```python
from build123d import *

# Parameters (mm, degrees)
F0_W     = 117
F0_H     = 40
F0_W_2   = 2
F1_DEPTH = 1.6
F2_DEPTH = 2.8
F3_W     = 119
F3_H     = 40
F3_W_2   = 115
F3_H_2   = 38
F4_DEPTH = 1
F6_DEPTH = 2
F8_DEPTH = 2


with BuildPart() as f1:
    # F0 (on Top) → F1 (new body)
    with BuildSketch(Plane.XY):
        with BuildLine():
            Line((62.5, 26), (-62.5, 26))
            ThreePointArc((-62.5, 26), (-63.914214, 25.414214), (-64.5, 24))
            Line((-64.5, 24), (-64.5, -24))
            ThreePointArc((-64.5, -24), (-63.914214, -25.414214), (-62.5, -26))
            Line((-62.5, -26), (62.5, -26))
            ThreePointArc((62.5, -26), (63.914214, -25.414214), (64.5, -24))
            Line((64.5, -24), (64.5, 24))
            ThreePointArc((64.5, 24), (63.914214, 25.414214), (62.5, 26))
        make_face()
        Polygon((60.5, 22), (60.5, 20), (60.5, -20), (60.5, -22), (-60.5, -22), (-60.5, 22), align=None, mode=Mode.SUBTRACT)
        Polygon((-58.5, -20), (-58.5, 20), (58.5, 20), (60.5, 20), (60.5, 22), (-60.5, 22), (-60.5, -22), (60.5, -22), (60.5, -20), (58.5, -20), align=None)
        Rectangle(F0_W, F0_H)
        with BuildLine():
            ThreePointArc((-56.5, 16), (-55.914214, 17.414214), (-54.5, 18))
            Line((-54.5, 18), (54.5, 18))
            ThreePointArc((54.5, 18), (55.914214, 17.414214), (56.5, 16))
            Line((56.5, 16), (56.5, -16))
            ThreePointArc((56.5, -16), (55.914214, -17.414214), (54.5, -18))
            Line((54.5, -18), (-54.5, -18))
            ThreePointArc((-54.5, -18), (-55.914214, -17.414214), (-56.5, -16))
            Line((-56.5, -16), (-56.5, 16))
        make_face(mode=Mode.SUBTRACT)
        with Locations((59.5, 0)):
            Rectangle(F0_W_2, F0_H)
    extrude(amount=-F1_DEPTH)

    # F0 (on Top) → F2 (join)
    with BuildSketch(Plane.XY):
        Polygon((-58.5, -20), (-58.5, 20), (58.5, 20), (60.5, 20), (60.5, 22), (-60.5, 22), (-60.5, -22), (60.5, -22), (60.5, -20), (58.5, -20), align=None)
    extrude(amount=F2_DEPTH)

    # F3 (on face) → F4 (join)
    with BuildSketch(Plane.XY.offset(2.8)):
        Polygon((60.5, 22), (-60.5, 22), (-60.5, -22), (60.5, -22), (60.5, -20), (-58.5, -20), (-58.5, 20), (60.5, 20), align=None)
        with Locations((1, 0)):
            Rectangle(F3_W, F3_H)
        Rectangle(F3_W_2, F3_H_2, mode=Mode.SUBTRACT)
    extrude(amount=F4_DEPTH)

    # F5 (on face) → F6 (join)
    with BuildSketch(Plane.XY.offset(3.8)):
        Polygon((-57.5, -19), (-57.5, 19), (57.5, 19), (58.5, 19), (58.5, 20), (-58.5, 20), (-58.5, -20), (58.5, -20), (58.5, -19), (57.5, -19), align=None)
    extrude(amount=F6_DEPTH)

    # F7 (on face) → F8 (join)
    with BuildSketch(Plane.XY.offset(5.8)):
        Polygon((-58.5, 20), (58.5, 20), (58.5, 21), (-59.5, 21), (-59.5, -21), (58.5, -21), (58.5, -20), (-58.5, -20), align=None)
        Polygon((-57.5, -19), (-57.5, 19), (57.5, 19), (58.5, 19), (58.5, 20), (-58.5, 20), (-58.5, -20), (58.5, -20), (58.5, -19), (57.5, -19), align=None)
    extrude(amount=F8_DEPTH)


solid = f1.part
```
Geometry check sheet. Reference: the model listing, model coordinates, mm. A direction names the side the tool comes from. Give positions to 0.01 mm unless a question says otherwise; leave off trailing zeros. Order: outer loops, then holes, each group sorted by start corner. A loop starts at its lowest first (then second) coordinate and runs counter-clockwise, first axis right, second up. Notation, with made-up numbers: (61.5, 65) - (97.5, 65) arc R30 ccw to (97.5, 102) - close; hole circle Ø4 at (88.25, -25). An arc over 180 degrees is marked (long way). Write item = value, one per line. Start each with the question number.
1) Section check B-B (x = -40.5). Enter the section's corners in (y, z), then the cut area to 3 significant figures.
2) Section check A-A (y = -6). Enter the section's corners in (x, z).
3) Draft check along X on faces 4 (the flat face through (-57.5, 0, 5)), 5 (the flat face through (2, -20, 1)), 6 (the flat face through (-60.5, 0, 2)). Enter one of: released by +X, released by -X, zero draft, split by the parting line, or undercut.
4) Gauge pin test, flat ends, axial feed: pin 1 Ø6 at (x, y) = (31.5, -12.5) entering from +Z; pin 2 Ø2 at (y, z) = (-2.5, 5) entering from -X; pin 3 Ø1.1 at (x, z) = (29, 2) entering from +Y; pin 4 Ø2 at (x, z) = (-8, 7) entering from -Y. Record the tip position at first contact, or that the pin passes through.
5) Scan lines: L1, parallel to Y at x = -37, z = 6.25; L2, parallel to Y at x = -19.5, z = 1.75; L3, parallel to X at y = -2, z = 3.5. Record each from-to range of solid material in increasing order.
6) Access from +Z, -Z, +X, -X, +Y, -Y to the whole of each face (thin tool, end or side, straight path). Record for faces 1 (the flat face through (-58.5, 0, 1)), 2 (the flat face through (-1, -22, 2)), 3 (the flat face through (0, 19, 5)).
Geometry check:
q1.outline = (-26, -1.6) - (-18, -1.6) - (-18, 0) - (-20, 0) - (-20, 2.8) - (-19, 2.8) - (-19, 7.8) - (-21, 7.8) - (-21, 5.8) - (-20, 5.8) - (-20, 3.8) - (-22, 3.8) - (-22, 0) - (-26, 0) - close; (18, -1.6) - (26, -1.6) - (26, 0) - (22, 0) - (22, 3.8) - (20, 3.8) - (20, 5.8) - (21, 5.8) - (21, 7.8) - (19, 7.8) - (19, 2.8) - (20, 2.8) - (20, 0) - (18, 0) - close
q1.area = 54.8 mm2
q2.outline = (-64.5, -1.6) - (-56.5, -1.6) - (-56.5, 0) - (-58.5, 0) - (-58.5, 2.8) - (-57.5, 2.8) - (-57.5, 7.8) - (-59.5, 7.8) - (-59.5, 5.8) - (-58.5, 5.8) - (-58.5, 3.8) - (-60.5, 3.8) - (-60.5, 0) - (-64.5, 0) - close; (56.5, -1.6) - (64.5, -1.6) - (64.5, 0) - (56.5, 0) - close; (57.5, 2.8) - (60.5, 2.8) - (60.5, 3.8) - (57.5, 3.8) - close
q3.face_4 = undercut
q3.face_5 = zero draft
q3.face_6 = released by -X
q4.pin_1 = through
q4.pin_2 = -59.5
q4.pin_3 = 22
q4.pin_4 = -21
q5.L1 = -21 to -19, 19 to 21
q5.L2 = -22 to -20, 20 to 22
q5.L3 = -60.5 to -57.5, 57.5 to 60.5
q6.face_1 = +X
q6.face_2 = +Z, +X, -X, -Y
q6.face_3 = +Z
